Model file for the job. Use its own axes, mm. Give positions to 0.01 mm unless a question says otherwise; leave off trailing zeros. Order: outer loops, then holes, each group sorted by start corner. A loop starts at its lowest first (then second) coordinate and runs counter-clockwise, first axis right, second up. Notation, with made-up numbers: (58, 65) -> (64, 65) arc R15 cw to (64, 83) -> close; hole circle Ø1 at (-22, 13.25). An arc over 180 degrees is marked (long way). Answer in a Markdown table with one row per item. Add a question column.
from build123d import *

# Parameters (mm, degrees)
SKETCH1_R           = 2.5
BOSS_EXTRUDE1_DEPTH = 3


with BuildPart() as part:
    # Sketch1 → Boss-Extrude1 (new body)
    with BuildSketch(Plane(origin=(0, 0, 0), x_dir=(1, 0, 0), z_dir=(0, 1, 0))):
        Polygon((-105, -11.825), (-75, -11.825), (-75, -14.825), (-25, -14.825), (-25, -11.825), (25, -11.825), (25, -14.825), (75, -14.825), (75, -11.825), (105, -11.825), (105, 11.825), (75, 11.825), (75, 14.825), (25, 14.825), (25, 11.825), (-25, 11.825), (-25, 14.825), (-75, 14.825), (-75, 11.825), (-105, 11.825), align=None)
        with Locations(Location((-95, 5, 0), (0, 0, 270))):
            Circle(SKETCH1_R, mode=Mode.SUBTRACT)
        with Locations(Location((-95, -5, 0), (0, 0, 270))):
            Circle(SKETCH1_R, mode=Mode.SUBTRACT)
        with Locations(Location((95, 5, 0), (0, 0, 270))):
            Circle(SKETCH1_R, mode=Mode.SUBTRACT)
        with Locations(Location((95, -5, 0), (0, 0, 270))):
            Circle(SKETCH1_R, mode=Mode.SUBTRACT)
    extrude(amount=BOSS_EXTRUDE1_DEPTH)


solid = part.part
Item 1: Wall check: line 1 (X direction, y = 0.7, z = 5); line 2 (X direction, y = 0.45, z = 7); line 3 (X direction, y = 1.15, z = -13.25). Give the ranges that are in metal, low to high.
Item 2: Saw through at C-C on y = 1.4. List the corners of the cut face in (x, z) (3 decimals).
Item 3: Saw through at B-B on z = 5. List the corners of the cut face in (x, y), plus the area to 3 significant figures.
Item 4: Two-plate mould, pull along X, no slides. Class faces 1 (the flat face through (-1, 3, 0)), 2 (the cylindrical face through (-92.52, 1.48, 4.67)): pulls with the +X half, pulls with the -X half, needs draft (parallel to the pull), parting line crosses it, or undercut.
Item 5: Pin check, flat tips, straight feed: pin 1 Ø0.9 at (y, z) = (1.5, 13) entering from +X; pin 2 Ø1.5 at (x, y) = (-8, 1.5) entering from -Z (3 decimals); pin 3 Ø8 at (x, z) = (31, -3) entering from -Y; pin 4 Ø0.9 at (y, z) = (2, -13.5) entering from -X. Stop position of each tip, or through.
Item 6: Saw through at A-A on x = 95. List the corners of the cut face in (y, z) (3 decimals).
Evaluation:
| question | item | result |
|---|---|---|
| 1 | line 1 | x = -105 to -97.5, -92.5 to 92.5, 97.5 to 105 |
| 1 | line 2 | x = -105 to -96.5, -93.5 to 93.5, 96.5 to 105 |
| 1 | line 3 | x = -75 to -25, 25 to 75 |
| 2 | outline | (-105, -11.825) -> (-75, -11.825) -> (-75, -14.825) -> (-25, -14.825) -> (-25, -11.825) -> (25, -11.825) -> (25, -14.825) -> (75, -14.825) -> (75, -11.825) -> (105, -11.825) -> (105, 11.825) -> (75, 11.825) -> (75, 14.825) -> (25, 14.825) -> (25, 11.825) -> (-25, 11.825) -> (-25, 14.825) -> (-75, 14.825) -> (-75, 11.825) -> (-105, 11.825) -> close; hole circle Ø5 at (-95, -5); hole circle Ø5 at (-95, 5); hole circle Ø5 at (95, -5); hole circle Ø5 at (95, 5) |
| 3 | outline | (-105, 0) -> (-97.5, 0) -> (-97.5, 3) -> (-105, 3) -> close; (-92.5, 0) -> (92.5, 0) -> (92.5, 3) -> (-92.5, 3) -> close; (97.5, 0) -> (105, 0) -> (105, 3) -> (97.5, 3) -> close |
| 3 | area | 600 mm2 |
| 4 | face 1 | needs draft |
| 4 | face 2 | undercut |
| 5 | pin 1 | stops at x = 75 |
| 5 | pin 2 | stops at z = -11.825 |
| 5 | pin 3 | stops at y = 0 |
| 5 | pin 4 | stops at x = -75 |
| 6 | outline | (0, -11.825) -> (3, -11.825) -> (3, -7.5) -> (0, -7.5) -> close; (0, -2.5) -> (3, -2.5) -> (3, 2.5) -> (0, 2.5) -> close; (0, 7.5) -> (3, 7.5) -> (3, 11.825) -> (0, 11.825) -> close |
